Model file for the job. Use its own axes, mm. Coordinates: 2 decimals unless noted, no trailing zeros. Write each loop counter-clockwise with the first axis right and the second up, starting at its lowest first coordinate (ties: lowest second). Pieces come first, ordered by that corner, then holes. Notation, with made-up numbers: M 88,-17.5 L 96,-17.5 A15 ccw 96,1.5 Z; hole C 13.5,1 d4. An arc over 180 degrees is marked long. Put each result on its own line as item: value. Start each with the question number.
Q1. Drill centre lines: line 1 along X through (y, z) = (278.5, 34); line 2 along X through (y, z) = (265.5, 4); line 3 along Y through (x, z) = (321, 67). Where is each one in solid material? Low to high.
Q2. Pull direction X, two halves, no side cores. Call faces 1 (the cylindrical face through (94.84, 339.44, 37.57)), 2 (the cylindrical face through (96.696, 342.119, 37.567)): pulls with the +X half, pulls with the -X half, needs draft (parallel to the pull), parting line crosses it, or undercut.
Q3. Drop flat-ended pins along their axis: pin 1 (12 mm diameter, centred on x = 166, z = 34, fed in from +Y); pin 2 (3 mm diameter, centred on x = 180.5, z = 15, fed in from +Y); pin 3 (5 mm diameter, centred on x = 209, z = 63.5, fed in from +Y). Give the stop position or say it passes through.
Q4. Cut at A-A (y = 323.5). Write the cut outline in (x, z).
Q5. Cut at C-C (x = 274.5). Write the cut outline in (y, z), then the cut area to 3 significant figures.
Q6. Cut at B-B (z = 69.5). Write the cut outline in (x, y).
Autodesk Inventor part; units mm, degrees
ref_plane "Work Plane3" through (373.5188, 62.0926, 0) normal (0.9729, 0.2313, 0) x (-0.2313, 0.9729, 0)
ref_plane "Work Plane4" through (-271.6172, 233.6803, 0) normal (-0.7295, 0.684, 0) x (-0.684, -0.7295, 0)
ref_plane "YZ Plane" through (0, 0, 0) normal (1, 0, 0) x (0, 1, 0)
sketch "Sketch1" plane through (0, 0, 0) normal (0, 0, 1) x (1, 0, 0)
  arc A0 (370.2866, 62.5027) -> (-270.1768, 230.7579) centre (4.8231, -25.5444) ccw
  arc A1 (373.5188, 62.0926) -> (-271.6172, 233.6803) centre (4.8231, -25.5444) ccw
  line L0 (-271.6172, 233.6803) -> (-270.1768, 230.7579)
  line L1 (370.2866, 62.5027) -> (373.5188, 62.0926)
  point P0 (0, 0)
  dimension "d0" = 375.92
  dimension "d1" = 123.47
  dimension "d3" = 123.47
  dimension "d4" = 378.968
extrude "Extrusion1" add sketch "Sketch1" along normal blind 76.2
ref_plane "Work Plane3" through (373.5188, 62.0926, 0) normal (0.9729, 0.2313, 0) x (-0.2313, 0.9729, 0)
ref_plane "Work Plane4" through (-271.6172, 233.6803, 0) normal (-0.7295, 0.684, 0) x (-0.684, -0.7295, 0)
sketch "Sketch2" plane through (373.5188, 62.0926, 0) normal (0.9729, 0.2313, 0) x (-0.2313, 0.9729, 0)
  line L0 (316.1255, 76.2) -> (0, 76.2)
  line L1 (0, 0) -> (0, 76.2)
  line L2 (316.1255, 0) -> (0, 0)
  line L3 (316.1255, 0) -> (316.1255, 76.2)
  point P0 (25.9674, 0)
  point P1 (38.1, 57.15)
  point P2 (38.1, 38.1)
  point P3 (38.1, 19.05)
  dimension "d7" = 38.1
  dimension "d8" = 38.1
  dimension "d9" = 38.1
  dimension "d10" = 19.05
  dimension "d11" = 38.1
  dimension "d12" = 57.15
sketch "Sketch3" plane through (-271.6172, 233.6803, 0) normal (-0.7295, 0.684, 0) x (-0.684, -0.7295, 0)
  line L0 (0, 0) -> (0, 76.2)
  line L1 (-378.968, 0) -> (0, 0)
  point P0 (-15.3344, 0)
  point P1 (-38.1, 19.05)
  point P2 (-38.1, 38.1)
  point P3 (-38.1, 57.15)
  point P4 (-316.1255, 0)
  dimension "d13" = 38.1
  dimension "d14" = 38.1
  dimension "d15" = 38.1
  dimension "d16" = 19.05
  dimension "d17" = 38.1
  dimension "d18" = 57.15
hole "Hole1" at (-245.5557, 261.4726, 57.15) at (-245.5557, 261.4726, 38.1) at (-245.5557, 261.4726, 19.05) direction (0.7295, -0.684, 0) diameter 6.35 depth 25.4 tip angle 118
hole "Hole2" at (364.7081, 99.1598, 57.15) at (364.7081, 99.1598, 38.1) at (364.7081, 99.1598, 19.05) direction (-0.9729, -0.2313, 0) diameter 6.35 depth 25.4 tip angle 118
thread "Thread7"
thread "Thread8"
thread "Thread9"
thread "Thread10"
thread "Thread11"
thread "Thread12"
equation "\"d3\" = d1"
properties part number "curvedTrack 123.47 degrees"
Computed values:
1. line 1: -221.39 to -216.25, 225.9 to 231.04
1. line 2: -237.89 to -233.1, 242.75 to 247.54
1. line 3: 177.8 to 183.38
2. face 1: undercut
2. face 2: parting line crosses it
3. pin 1: y = 320.2
3. pin 2: y = 311.03
3. pin 3: y = 295.3
4. outline: M -142.77,0 L -134.76,0 L -134.76,76.2 L -142.77,76.2 Z; M 144.41,0 L 152.42,0 L 152.42,76.2 L 144.41,76.2 Z
5. outline: M 236.35,0 L 240.71,0 L 240.71,76.2 L 236.35,76.2 Z
5. area: 332 mm2
6. outline: M -271.62,233.68 L -270.18,230.76 A375.92 cw 370.29,62.5 L 373.52,62.09 A378.97 ccw Z
